```python
from build123d import *

# Parameters (mm, degrees)
F1_DEPTH       = 22
F3_R           = 10
F4_DEPTH       = 6
F6_DEPTH       = 20
F7_W           = 10
F7_H           = 10
F8_DEPTH       = 55.001
F8_DEPTH_BACK  = 15.001
F9_W           = 40
F9_H           = 30
F10_DEPTH      = 15
F10_DEPTH_BACK = 55
F2_W           = 40
F2_H           = 10
F11_DEPTH      = 40


# Not quite as in the source:
# - an extrude ends at something that could not be found from the text; its depth is read off the source's solid


with BuildPart() as f1:
    # F0 (on Top) → F1 (new body)
    with BuildSketch(Plane.XY):
        with BuildLine():
            Line((40, 18.5987265639), (0, 18.5987265639))
            Line((0, 18.5987265639), (0, -21.4012734361))
            ThreePointArc((0, -21.4012734361), (20, -41.4012734361), (40, -21.4012734361))
            Line((40, -21.4012734361), (40, 18.5987265639))
        make_face()
    extrude(amount=F1_DEPTH)

    # F3 (on face) → F4 (cut)
    with BuildSketch(Plane.XY.offset(22)):
        with Locations((20, -21.4012734361)):
            Circle(F3_R)
    extrude(amount=-F4_DEPTH, mode=Mode.SUBTRACT)

    # F5 (on face) → F6 (join)
    with BuildSketch(Plane(origin=(0, 0, 0), x_dir=(1, 0, 0), z_dir=(0, 0, -1))):
        Polygon((0, 55.4012734361), (-15, 21.4012734361), (55, 21.4012734361), (40, 55.4012734361), align=None)
    extrude(amount=F6_DEPTH)

    # F7 (on face) → F8 (cut, two sides)
    with BuildSketch(Plane.YZ.offset(40)) as f8_sk:
        with Locations((-50.4012734361, -5)):
            Rectangle(F7_W, F7_H)
    extrude(amount=-F8_DEPTH, mode=Mode.SUBTRACT)
    extrude(f8_sk.sketch, amount=F8_DEPTH_BACK, mode=Mode.SUBTRACT)

    # F9 (on face) → F10 (join, two sides)
    with BuildSketch(Plane.YZ.offset(40)) as f10_sk:
        with Locations((-1.4012734361, -5)):
            Rectangle(F9_W, F9_H)
    extrude(amount=F10_DEPTH)
    extrude(f10_sk.sketch, amount=-F10_DEPTH_BACK)

    # F2 (on face) → F11 (cut, through all)
    with BuildSketch(Plane.YZ.offset(40)):
        with Locations((-21.4012734361, 11)):
            Rectangle(F2_W, F2_H)
    extrude(amount=-F11_DEPTH, mode=Mode.SUBTRACT)


solid = f1.part
```
The model under review builds one solid part; all positions refer to its coordinate system, in mm. A direction names the side the tool comes from. Round coordinates to 2 decimals unless told otherwise and drop trailing zeros. Write each loop counter-clockwise with the first axis right and the second up, starting at its lowest first coordinate (ties: lowest second). Pieces come first, ordered by that corner, then holes. Notation, with made-up numbers: M 32.5,27.5 L 53.5,27.5 A13 ccw 53.5,49.5 Z; hole C 55,85 d1. An arc over 180 degrees is marked long. Use CSV: the item, a comma, the result in double quotes. Start each with the question number.
(1) The part is to be moulded in two halves that separate along Z. For faces 4 (the face through (20, -8, 16)), 5 (the face through (-9, -35, -10)), 6 (the face through (20, -19, -20)), 7 (the face through (20, -1.401, 11)), say which applies: +Z half, -Z half, draft (parallel to the pull), parting line (faces both ways), or undercut.
(2) We need section B-B, the plane y = 1.5. State the section outline as (x, z) points.
(3) Tool access review of faces 1 (the face through (-7, -21.401, 5)), 2 (the face through (40, 3, 17)), 3 (the face through (-7, -2, 10)): name each direction out of +Z, -Z, +X, -X, +Y, -Y from which nothing blocks a thin tool from reaching the whole face with its end or side.
(4) For line 1 along Z through (x, y) = (30, -7); line 2 along Y through (x, z) = (20, 19.6); line 3 along Y through (x, z) = (-9.5, 4), list the stretches that pass through material, from the lowest coordinate up.
(5) We need section C-C, the plane y = -14. State the section outline as (x, z) points.
(6) We need section A-A, the plane x = 20. State the section outline as (y, z) points.
(7) We need section D-D, the plane z = -9. State the section outline as (x, y) points, then the cut area to 3 significant figures.
(8) Clearance check with flat-ended pins moving along their axes: P1, Ø1.5, axis at y = -33.5, z = 17.5, coming from the -X side; P2, Ø6, axis at y = -11.5, z = 13.5, coming from the -X side; P3, Ø6, axis at y = -7.5, z = 16, coming from the +X side. State where each tip first meets the part, or that it passes through.
Findings:
1,face 4,"undercut"
1,face 5,"draft"
1,face 6,"-Z half"
1,face 7,"undercut"
2,outline,"M -15,-20 L 55,-20 L 55,10 L 40,10 L 40,22 L 0,22 L 0,10 L -15,10 Z"
3,face 1,"+Z, -X, -Y"
3,face 2,"+Z, +X, +Y, -Y"
3,face 3,"+Z, -X, +Y, -Y"
4,line 1,"-20 to 6, 16 to 22"
4,line 2,"-41.4 to -31.4, -11.4 to 18.6"
4,line 3,"-21.4 to 18.6"
5,outline,"M -15,-20 L 55,-20 L 55,10 L 40,10 L 40,6 L 0,6 L 0,10 L -15,10 Z; M 0,16 L 13.28,16 L 13.28,22 L 0,22 Z; M 26.72,16 L 40,16 L 40,22 L 26.72,22 Z"
6,outline,"M -55.4,-20 L 18.6,-20 L 18.6,22 L -11.4,22 L -11.4,16 L -1.4,16 L -1.4,6 L -41.4,6 L -41.4,0 L -45.4,0 L -45.4,-10 L -55.4,-10 Z; M -41.4,16 L -31.4,16 L -31.4,22 L -41.4,22 Z"
7,outline,"M -15,-21.4 L -4.41,-45.4 L 44.41,-45.4 L 55,-21.4 L 55,18.6 L -15,18.6 Z"
7,area,"4,230 mm^2"
8,P1,"x = 3.53"
8,P2,"x = 0"
8,P3,"x = 40"
